```python
from build123d import *

# Parameters (mm, degrees)
SKETCH1_W           = 158
SKETCH1_H           = 92
BOSS_EXTRUDE1_DEPTH = 8
SKETCH2_W           = 158
SKETCH2_H           = 92
SKETCH2_W_2         = 148
SKETCH2_H_2         = 82
BOSS_EXTRUDE2_DEPTH = 15
SKETCH3_R           = 33
CUT_EXTRUDE1_DEPTH  = 95.265582266
FILLET1_R           = 5
FILLET2_R           = 5


with BuildPart() as part:
    # Sketch1 → Boss-Extrude1 (new body)
    with BuildSketch(Plane(origin=(0, 0, 0), x_dir=(1, 0, 0), z_dir=(0, 1, 0))):
        Rectangle(SKETCH1_W, SKETCH1_H)
    extrude(amount=BOSS_EXTRUDE1_DEPTH)

    # Sketch2 → Boss-Extrude2 (add)
    with BuildSketch(Plane(origin=(0, 8, 0), x_dir=(1, 0, 0), z_dir=(0, 1, 0))):
        Rectangle(SKETCH2_W, SKETCH2_H)
        Rectangle(SKETCH2_W_2, SKETCH2_H_2, mode=Mode.SUBTRACT)
    extrude(amount=BOSS_EXTRUDE2_DEPTH)

    # Sketch3 → Cut-Extrude1 (cut, through all)
    with BuildSketch(Plane.XZ):
        with Locations(Location((0, 0, 0), (0, 0, 270))):
            Circle(SKETCH3_R)
    extrude(amount=-CUT_EXTRUDE1_DEPTH, mode=Mode.SUBTRACT)

    # Fillet1
    fillet1_edges = [part.edges().sort_by_distance(p)[0] for p in [
        (-79, 11.5, 46),
    ]]
    fillet(fillet1_edges, radius=FILLET1_R)

    # Fillet2
    fillet2_edges = [part.edges().sort_by_distance(p)[0] for p in [
        (79, 11.5, 46),
        (-79, 11.5, -46),
        (79, 11.5, -46),
    ]]
    fillet(fillet2_edges, radius=FILLET2_R)


solid = part.part
```
Can you work these out from the model? Positions are in its coordinate system, mm. A direction names the side the tool comes from. Give positions to 0.01 mm unless a question says otherwise; leave off trailing zeros. Loops run counter-clockwise (first coordinate to the right, second up) from the corner with the lowest first, then second, coordinate; pieces in that order, holes last. Notation, with made-up numbers: M 73.5,47.5 L 90.5,47.5 A14 ccw 90.5,52.5 Z; hole C -9,56.25 d1. An arc over 180 degrees is marked long. One line per question, with ' | ' between items. Start each with the question number.
Q1. If we mould it in two halves opening along Z, with no side actions, what happens to faces 3 (the cylindrical face through (77, 12, 45)), 4 (the flat face through (79, 11, 1)), 5 (the flat face through (-1, 15, -41))? For each: +Z half, -Z half, draft (parallel to the pull), parting line (faces both ways), or undercut.
Q2. If we section it at D-D (y = 11): Please give me the cut outline in (x, z).
Q3. For faces 1 (the flat face through (74, 15, 1)), 2 (the flat face through (-36, 0, -1)), which set-ups out of +Z, -Z, +X, -X, +Y, -Y let a thin tool reach every point of the face, with its end or its side?
Q4. If I drill on line 1 (Z direction, x = -59.5, y = 13.25); line 2 (X direction, y = 2.25, z = 0); line 3 (X direction, y = 12.5, z = -4.5), over which ranges is the centre line in solid material (lowest first)? Write a range as from..to.
Q5. If we section it at A-A (z = 0): Please give me the cut outline in (x, y), plus the area to 3 significant figures.
Q6. If we section it at B-B (x = 0): Please give me the cut outline in (y, z), plus the area to 3 significant figures.
Q7. For pin 1 Ø5 at (x, z) = (-57.5, -9) entering from +Y, with a flat end and sliding along its axis, tell me the tip position at first contact or that it passes through.
Q8. If we section it at C-C (y = 4): Please give me the cut outline in (x, z).
Computed:
1) face 3: +Z half | face 4: draft | face 5: undercut
2) outline: M -79,-41 A5 ccw -74,-46 L 74,-46 A5 ccw 79,-41 L 79,41 A5 ccw 74,46 L -74,46 A5 ccw -79,41 Z; hole M -74,-41 L 74,-41 L 74,41 L -74,41 Z
3) face 1: +Y | face 2: +Z, -Z, +X, -X, -Y
4) line 1: z = -46..-41, 41..46 | line 2: x = -79..-33, 33..79 | line 3: x = -79..-74, 74..79
5) outline: M -79,0 L -33,0 L -33,8 L -74,8 L -74,23 L -79,23 Z; M 33,0 L 79,0 L 79,23 L 74,23 L 74,8 L 33,8 Z | area: 886 mm²
6) outline: M 0,-46 L 23,-46 L 23,-41 L 8,-41 L 8,-33 L 0,-33 Z; M 0,33 L 8,33 L 8,41 L 23,41 L 23,46 L 0,46 Z | area: 358 mm²
7) pin 1: stops at y = 8
8) outline: M -79,-41 A5 ccw -74,-46 L 74,-46 A5 ccw 79,-41 L 79,41 A5 ccw 74,46 L -74,46 A5 ccw -79,41 Z; hole C 0,0 d66
